```python
from build123d import *

# Parameters (mm, degrees)
SKETCH_1_R          = 14
SKETCH_2_R          = 18
SKETCH_2_R_2        = 2
EXTRUDE_2_DEPTH     = 5
SKETCH_3_R          = 3
CUT_EXTRUDE_1_DEPTH = 20


with BuildPart() as part:
    # 草图1 → 旋转1 (revolve)
    with BuildSketch(Plane(origin=(0, 0, 0), x_dir=(0, 0, -1), z_dir=(1, 0, 0))):
        with Locations((0, 30)):
            Circle(SKETCH_1_R)
    revolve(axis=Axis((0, 0, 15.4), (0, 0, -1)))

    # 草图2 → 凸台-拉伸2 (add, symmetric)
    with BuildSketch(Plane.XY):
        Circle(SKETCH_2_R)
        Circle(SKETCH_2_R_2, mode=Mode.SUBTRACT)
    extrude(amount=EXTRUDE_2_DEPTH, both=True)

    # 草图3 → 切除-拉伸1 (cut, through all)
    with BuildSketch(Plane.XY.offset(5)):
        with Locations((0, 10)):
            Circle(SKETCH_3_R)
        with Locations((7.071067812, 7.071067812)):
            Circle(SKETCH_3_R)
        with Locations((10, 0)):
            Circle(SKETCH_3_R)
        with Locations((7.071067812, -7.071067812)):
            Circle(SKETCH_3_R)
        with Locations((0, -10)):
            Circle(SKETCH_3_R)
        with Locations((-7.071067812, -7.071067812)):
            Circle(SKETCH_3_R)
        with Locations((-10, 0)):
            Circle(SKETCH_3_R)
        with Locations((-7.071067812, 7.071067812)):
            Circle(SKETCH_3_R)
    extrude(amount=-CUT_EXTRUDE_1_DEPTH, mode=Mode.SUBTRACT)


solid = part.part
```
The listing builds one solid part. Answer for the finished solid, in the listing's coordinates (mm). A direction names the side the tool comes from. Coordinates: 2 decimals unless noted, no trailing zeros. Loops run counter-clockwise (first coordinate to the right, second up) from the corner with the lowest first, then second, coordinate; pieces in that order, holes last. Notation, with made-up numbers: (21, -2) -> (47, -2) arc R8 ccw to (47, 8) -> close; hole circle Ø4 at (-16, 22). An arc over 180 degrees is marked (long way). Return JSON: item names as keys, results as strings. Group by question number.
(1) A cutting plane is placed at A-A on x = 0. Write down the section's boundary in (y, z), and give its area (3 significant figures).
(2) Given pin 1 Ø9.5 at (x, y) = (0, -10) entering from -Z; pin 2 Ø1 at (x, y) = (-32.5, -28.5) entering from -Z; pin 3 Ø2 at (x, y) = (-11, -9) entering from +Z; pin 4 Ø12 at (x, z) = (-3, 4.5) entering from +Y, each flat-ended and moving along its own axis, determine where each tip first touches the part or whether it passes through.
(3) Which of the six approach directions +Z, -Z, +X, -X, +Y, -Y give full straight-line access (tool end or side, diameter ignored) to faces 1 (the flat face through (0, -4, -5)), 2 (the cylindrical face through (-3, 10, 0)), 3 (the flat face through (0, -4, 5))?
(4) Find the intervals of material crossed by probe 1 along Y at (x, z) = (8, 4.5); probe 2 along Z at (x, y) = (-1, -14.5); probe 3 along X at (y, z) = (-3.5, 8), in increasing order. Write a range as from..to.
(5) A cutting plane is placed at C-C on z = -0.5. Count the separate pieces of the cut face and the enclosed holes in it, and give its area (3 significant figures).
(6) A cutting plane is placed at D-D on z = -10.25. Write down the section's boundary in (x, y).
The answers:
{
 "1": {"outline": "(-16.92, -5) -> (-13, -5) -> (-13, 5) -> (-16.92, 5) arc R14 ccw (long way) to start; (-7, -5) -> (-2, -5) -> (-2, 5) -> (-7, 5) -> close; (2, -5) -> (7, -5) -> (7, 5) -> (2, 5) -> close; (13, -5) -> (16.92, -5) arc R14 ccw (long way) to (16.92, 5) -> (13, 5) -> close", "area": "1,400 mm^2"},
 "2": {"pin 1": "stops at z = -5", "pin 2": "stops at z = -5.83", "pin 3": "stops at z = 5", "pin 4": "stops at y = 44"},
 "3": {"face 1": "-Z", "face 2": "+Z, -Z", "face 3": "+Z"},
 "4": {"probe 1": "y = -42.51..-9.92, -4.22..-2.24, 2.24..4.22, 9.92..42.51", "probe 2": "z = -5..5", "probe 3": "x = -41.34..-18.18, 18.18..41.34"},
 "5": {"separate pieces": "1", "enclosed holes": "9", "area": "5,840 mm^2"},
 "6": {"outline": "circle Ø79.07 at (0, 0); hole circle Ø40.93 at (0, 0)"}
}
